The model under review builds one solid part; all positions refer to its coordinate system, in mm. A direction names the side the tool comes from. Round coordinates to 2 decimals unless told otherwise and drop trailing zeros. Write each loop counter-clockwise with the first axis right and the second up, starting at its lowest first coordinate (ties: lowest second). Pieces come first, ordered by that corner, then holes. Notation, with made-up numbers: (22.5, 74.25) - (30.5, 74.25) arc R16 ccw to (30.5, 81.25) - close; hole circle Ø4 at (32.5, 89). An arc over 180 degrees is marked (long way). Use one line per item in the form item = value.
from build123d import *

# Parameters (mm, degrees)
SKETCH2_W           = 20
SKETCH2_H           = 15
BOSS_EXTRUDE1_DEPTH = 5
SKETCH3_W           = 5
SKETCH3_H           = 15
BOSS_EXTRUDE2_DEPTH = 50
FILLET1_R           = 0.5
FILLET2_R           = 0.5


with BuildPart() as part:
    # Sketch2 → Boss-Extrude1 (new body)
    with BuildSketch(Plane(origin=(0, 0, 0), x_dir=(1, 0, 0), z_dir=(0, 1, 0))):
        with Locations((10, 7.5)):
            Rectangle(SKETCH2_W, SKETCH2_H)
    extrude(amount=BOSS_EXTRUDE1_DEPTH)

    # Sketch3 → Boss-Extrude2 (add)
    with BuildSketch(Plane(origin=(0, 5, 0), x_dir=(1, 0, 0), z_dir=(0, 1, 0))):
        with Locations((17.5, 7.5)):
            Rectangle(SKETCH3_W, SKETCH3_H)
    extrude(amount=BOSS_EXTRUDE2_DEPTH)

    # Fillet1
    fillet1_edges = [part.edges().sort_by_distance(p)[0] for p in [
        (20, 0, -7.5),
    ]]
    fillet(fillet1_edges, radius=FILLET1_R)

    # Fillet2
    fillet2_edges = [part.edges().sort_by_distance(p)[0] for p in [
        (15, 5, -7.5),
    ]]
    fillet(fillet2_edges, radius=FILLET2_R)


solid = part.part
(1) Machinability: for faces 1 (the flat face through (7, 5, -8)), 2 (the flat face through (10, 0, -8)), which of the approach directions +Z, -Z, +X, -X, +Y, -Y give a long, thin tool a straight path to every point of the face, cutting with its end or side? Answer none if there is none.
Geometry results:
face_1 = +Z, -Z, -X, +Y
face_2 = +Z, -Z, +X, -X, -Y
(2) Add section B-B on y = 15.5. Write out the cut boundary in (x, z), then the cut area to 3 significant figures.
Geometry results:
outline = (15, -15) - (20, -15) - (20, 0) - (15, 0) - close
area = 75.0 mm2
(3) Insertion check: P1, Ø4.5, axis at x = 5, z = -4, coming from the +Y side. The pin has a flat end and moves straight along its axis. Give the tip position at first contact, or say it passes through.
Geometry results:
P1 = 5
(4) Add section A-A on z = -5.25. Write out the cut boundary in (x, y).
Geometry results:
outline = (0, 0) - (19.5, 0) arc R0.5 ccw to (20, 0.5) - (20, 55) - (15, 55) - (15, 5.5) arc R0.5 cw to (14.5, 5) - (0, 5) - close
(5) Add section C-C on x = 7.75. Write out the cut boundary in (y, z).
Geometry results:
outline = (0, -15) - (5, -15) - (5, 0) - (0, 0) - close
(6) To check wall thickness, follow L1, parallel to Y at x = 13.25, z = -2.75; L2, parallel to X at y = 26.5, z = -1.5. State the ranges of each line that lie inside material, in increasing order.
Geometry results:
L1 = 0 to 5
L2 = 15 to 20
